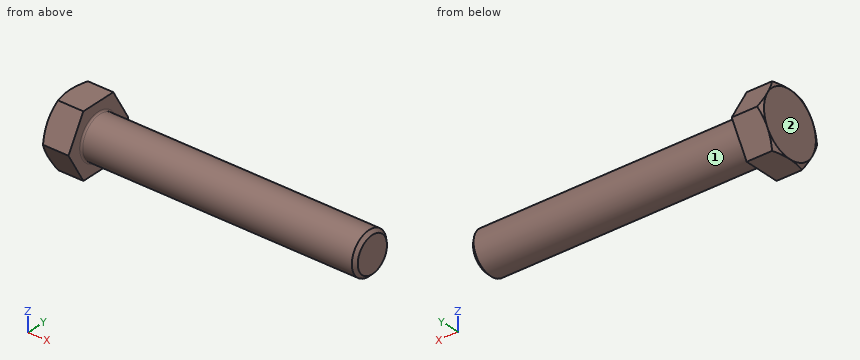
Autodesk Inventor part; units mm, degrees
ref_plane "Work Plane1" through (1.525, 0, 0) normal (0, 0, 1) x (1, 0, 0)
ref_plane "YZ Plane" through (0, 0, 0) normal (1, 0, 0) x (0, 1, 0)
ref_plane "XZ Plane" through (0, 0, 0) normal (0, 1, 0) x (-1, 0, 0)
sketch "Sketch1" plane through (0, 0, 0) normal (0, 0, 1) x (1, 0, 0)
  line L0 (0, 10) -> (130, 10)
  line L1 (130, 10) -> (130, 0)
  line L2 (130, 0) -> (0, 0)
  line L3 (-26, 0) -> (156, 0)
  line L4 (0, -2) -> (0, 12)
  line L5 (0, 10) -> (0, 0)
  dimension "d2" = 20
  dimension "d59" = 130
revolve "Body" add sketch "Sketch1" angle 360 about axis through (130, 0, 0) along (-1, 0, 0)
sketch "Sketch2" plane through (0, 0, 0) normal (-1, 0, 0) x (0, 0, 1)
  line L0 (0, 17.3205) -> (15, 8.6603)
  line L1 (15, 8.6603) -> (15, -8.6603)
  line L2 (15, -8.6603) -> (0, -17.3205)
  line L3 (0, -17.3205) -> (-15, -8.6603)
  line L4 (-15, -8.6603) -> (-15, 8.6603)
  line L5 (-15, 8.6603) -> (0, 17.3205)
  line L6 (-21, 0) -> (21, 0)
  line L7 (0, 24.2487) -> (0, -24.2487)
  point P0 (0, 0)
  point P1 (0, 0)
  dimension "d11" = 30
extrude "Head" add sketch "Sketch2" along normal blind 13.4
sketch "Sketch4" plane through (0, 0, 0) normal (0, 0, 1) x (1, 0, 0)
  line L0 (-11.6679, 18) -> (-13.4, 15)
  line L1 (-1.1, 0) -> (-0.234, 0)
  line L2 (-16.0332, 0) -> (2.3992, 0)
  line L3 (-13.4, 18) -> (-11.6679, 18)
  line L4 (-13.4, 15) -> (-13.4, 18)
  line L5 (0, 21.6) -> (0, -3.6)
  dimension "d65" = 30
  dimension "d67" = 30
  dimension "d68" = 36
  dimension "d69" = 13.4
revolve "Chamfer1" cut sketch "Sketch4" angle 360 about axis through (-1.1, 0, 0) along (1, 0, 0)
thread "Thread"
chamfer "Chamfer2" distance 1.5336 distance2 1.5337 1 edges at (130, -10, 0) measured on face at (130, -2.6738, -2.9356)
fillet "Fillet" radius 0.8 1 edges at (0, -10, 0)
ref_plane "Work Plane1" through (1.525, 0, 0) normal (0, 0, 1) x (1, 0, 0)
equation "\"d2\" = GD"
equation "\"d59\" = NLG"
equation "\"d11\" = SW"
equation "\"d3\" = KOH"
equation "\"d15\" = GEL"
equation "\"d6\" = -0.5 * SPD + 0.5 * GD"
equation "\"d71\" = RR1"
equation "\"d65\" = SW"
equation "\"d67\" = ANG1"
equation "\"d68\" = 1.2 * SW"
equation "\"d69\" = KOH"
equation "\"NLG\" = 130"
equation "\"GD\" = NND"
equation "\"KOH\" = 13.4"
equation "\"GEL\" = 52"
equation "\"SW\" = 30"
equation "\"SPD\" = NND - 1.2269 * PTC"
equation "\"SD\" = 0"
equation "\"ANG1\" = 30deg"
equation "\"GAL\" = 0.61345 * PTC"
equation "\"GUL\" = 0.61345 * PTC"
equation "\"RR\" = 0.1"
equation "\"RR1\" = 0.8"
equation "\"GD1\" = THREADDIA - 1.2269 * PTC"
equation "\"TOA\" = 30deg"
equation "\"PTC\" = 2.5"
equation "\"KOH1\" = 8.8"
equation "\"E0\" = 1.155 * SW"
properties part number "ANSI B18.2.3.5M - M20 x 2,5 x 130" material "Steel, Mild"
Geometry check sheet. Reference: the model listing, model coordinates, mm. Face numbers are marked on the shaded views. A direction names the side the tool comes from. Round coordinates to 2 decimals unless told otherwise and drop trailing zeros. Order: outer loops, then holes, each group sorted by start corner. A loop starts at its lowest first (then second) coordinate and runs counter-clockwise, first axis right, second up. Notation, with made-up numbers: (86, 5.5) - (116, 5.5) arc R27 cw to (116, 31.5) - close; hole circle Ø6 at (52.5, -25.5). An arc over 180 degrees is marked (long way). One line per question, with ' | ' between items. Start each with the question number.
(1) Sectioned sample at A-A on x = 101. Record the cut outline in (y, z), and give its area (3 significant figures).
(2) Thickness scan on L1, parallel to X at y = 11, z = 1; L2, parallel to Y at x = 115.5, z = -5. Record the ranges inside material, lowest first. Write a range as [from, to].
(3) Depth check by flat-ended pin: pin 1 Ø1.5 at (x, z) = (68, -3) entering from -Y; pin 2 Ø1 at (x, y) = (82.5, 6.5) entering from -Z; pin 3 Ø1.5 at (x, z) = (13.5, -0.5) entering from +Y. Enter the tip coordinate at first touch or a pass-through.
(4) Access from +Z, -Z, +X, -X, +Y, -Y to the whole of each face (thin tool, end or side, straight path). Record for the marked faces 1 and 2.
Conclusion:
1) outline: circle Ø20 at (0, 0) | area: 314 mm2
2) L1: x = [-13.4, 0] | L2: y = [-8.66, 8.66]
3) pin 1: stops at y = -9.74 | pin 2: stops at z = -8 | pin 3: stops at y = 10
4) face 1: +X | face 2: +Z, -Z, -X, +Y, -Y
